Input: part model. Units: mm. Frame: model coordinates. A direction names the side the tool comes from. Give positions to 0.01 mm unless a question says otherwise; leave off trailing zeros. Order: outer loops, then holes, each group sorted by start corner. A loop starts at its lowest first (then second) coordinate and runs counter-clockwise, first axis right, second up. Notation, with made-up numbers: (70, 53.25) - (97, 53.25) arc R15 ccw to (97, 76.25) - close; hole circle Ø7 at (-7.5, -3.75). An arc over 180 degrees is marked (long way). Answer in a Markdown table with one row per item. Add a question column.
1. Contact query for flat-ended pins moving along their axis: pin 1 (2 mm diameter, centred on x = 4, z = -63.5, fed in from -Y); pin 2 (1 mm diameter, centred on x = 3, z = -18.5, fed in from -Y) (3 decimals). Output: stop coordinate, or through.
2. Access query for faces 5 (the face through (3, 65.7, -40)), 6 (the face through (3, 120.7, -39)). Directions: +Z, -Z, +X, -X, +Y, -Y. A direction counts if a zero-diameter tool reaches every point of the face in a straight line with its end or side. Return the directions, or none.
3. Section query B-B on z = -39.75. Return loops of the section in (x, y), and give its area (3 significant figures).
4. Section query C-C on x = 2.55. Return loops of the section in (y, z), and give its area (3 significant figures).
5. Ray query, line 1 (Y direction, x = 1.5, z = -55); line 2 (Z direction, x = 5.7, y = 74); line 3 (Z direction, x = 3.35, y = 7). Return the intervals inside material, ascending. Write a range as [from, to].
6. Section query A-A on y = 36.35. Return loops of the section in (x, z).
7. Mould query, pull axis Z, two halves, no side actions, for faces 1 (the face through (3, 83, -42.25)), 2 (the face through (3, 0, -40)), 3 (the face through (3.042, 5.703, -73.486)), 4 (the face through (3, 100.7, -40)). Classes: released by +Z, released by -Z, zero draft, split by the parting line, or undercut.
```python
from build123d import *

# Parameters (mm, degrees)
BOSS_EXTRUDE2_DEPTH = 6
SKETCH2_W           = 5
SKETCH2_H           = 35
CUT_EXTRUDE1_DEPTH  = 10
SKETCH3_R           = 11
SKETCH3_R_2         = 1.5
CUT_EXTRUDE2_DEPTH  = 10
FILLET1_R           = 20


with BuildPart() as part:
    # Sketch1 → Boss-Extrude2 (new body)
    with BuildSketch(Plane(origin=(0, 0, 0), x_dir=(0, 0, -1), z_dir=(1, 0, 0))):
        Polygon((0, 43), (0, 120.7), (79.5, 120.7), (79.5, 43), (79.5, 0), (0, 0), align=None)
    extrude(amount=BOSS_EXTRUDE2_DEPTH)

    # Sketch2 → Cut-Extrude1 (cut)
    with BuildSketch(Plane(origin=(6, 0, 0), x_dir=(0, 0, -1), z_dir=(1, 0, 0))):
        with Locations((39.75, 83.2)):
            Rectangle(SKETCH2_W, SKETCH2_H)
    extrude(amount=-CUT_EXTRUDE1_DEPTH, mode=Mode.SUBTRACT)

    # Sketch3 → Cut-Extrude2 (cut)
    with BuildSketch(Plane(origin=(6, 0, 0), x_dir=(0, 0, -1), z_dir=(1, 0, 0))):
        with Locations((39.75, 21.1)):
            Circle(SKETCH3_R)
        with Locations((24.5, 36.35)):
            Circle(SKETCH3_R_2)
        with Locations((55, 36.35)):
            Circle(SKETCH3_R_2)
        with Locations((55, 5.85)):
            Circle(SKETCH3_R_2)
        with Locations((24.5, 5.85)):
            Circle(SKETCH3_R_2)
    extrude(amount=-CUT_EXTRUDE2_DEPTH, mode=Mode.SUBTRACT)

    # Fillet1
    fillet1_edges = [part.edges().sort_by_distance(p)[0] for p in [
        (3, 0, 0),
        (3, 0, -79.5),
    ]]
    fillet(fillet1_edges, radius=FILLET1_R)


solid = part.part
```
Answer:
| question | item | result |
|---|---|---|
| 1 | pin 1 | stops at y = 0.23 |
| 1 | pin 2 | stops at y = 0.025 |
| 2 | face 5 | +X, -X |
| 2 | face 6 | +Z, -Z, +X, -X, +Y |
| 3 | outline | (0, 0) - (6, 0) - (6, 10.1) - (0, 10.1) - close; (0, 32.1) - (6, 32.1) - (6, 65.7) - (0, 65.7) - close; (0, 100.7) - (6, 100.7) - (6, 120.7) - (0, 120.7) - close |
| 3 | area | 382 mm² |
| 4 | outline | (0, -59.5) arc R20 ccw to (20, -79.5) - (120.7, -79.5) - (120.7, 0) - (20, 0) arc R20 ccw to (0, -20) - close; hole circle Ø3 at (5.85, -55); hole circle Ø3 at (5.85, -24.5); hole circle Ø22 at (21.1, -39.75); hole circle Ø3 at (36.35, -55); hole circle Ø3 at (36.35, -24.5); hole (65.7, -42.25) - (100.7, -42.25) - (100.7, -37.25) - (65.7, -37.25) - close |
| 4 | area | 8,840 mm² |
| 5 | line 1 | y = [0, 4.35], [7.35, 34.85], [37.85, 120.7] |
| 5 | line 2 | z = [-79.5, -42.25], [-37.25, 0] |
| 5 | line 3 | z = [-74.7, -55.96], [-54.04, -25.46], [-23.54, -4.8] |
| 6 | outline | (0, -79.5) - (6, -79.5) - (6, -56.5) - (0, -56.5) - close; (0, -53.5) - (6, -53.5) - (6, -26) - (0, -26) - close; (0, -23) - (6, -23) - (6, 0) - (0, 0) - close |
| 7 | face 1 | undercut |
| 7 | face 2 | zero draft |
| 7 | face 3 | released by -Z |
| 7 | face 4 | undercut |
